```python
from build123d import *

# Parameters (mm, degrees)
SKETCH_1_W          = 42
SKETCH_1_H          = 8
SKETCH_1_R          = 2.35
EXTRUDE_1_DEPTH     = 32
SKETCH_2_W          = 23
SKETCH_2_H          = 20
CUT_EXTRUDE_2_DEPTH = 14
SKETCH_3_W          = 23
SKETCH_3_H          = 27.182471636
CUT_EXTRUDE_3_DEPTH = 10


with BuildPart() as part:
    # 草图1 → 凸台-拉伸1 (new, symmetric)
    with BuildSketch(Plane.XY):
        Rectangle(SKETCH_1_W, SKETCH_1_H)
        with Locations((-4.925, 0)):
            Circle(SKETCH_1_R, mode=Mode.SUBTRACT)
        with Locations(Location((4.925, 0, 0), (0, 0, 180))):
            Circle(SKETCH_1_R, mode=Mode.SUBTRACT)
        with Locations((-14.775, 0)):
            Circle(SKETCH_1_R, mode=Mode.SUBTRACT)
        with Locations(Location((14.775, 0, 0), (0, 0, 180))):
            Circle(SKETCH_1_R, mode=Mode.SUBTRACT)
    extrude(amount=EXTRUDE_1_DEPTH, both=True)

    # 草图2 → 切除-拉伸2 (cut)
    with BuildSketch(Plane(origin=(0, 4, 0), x_dir=(1, 0, 0), z_dir=(0, 1, 0))):
        with Locations((0, -15)):
            Rectangle(SKETCH_2_W, SKETCH_2_H)
        with Locations((0, 15)):
            Rectangle(SKETCH_2_W, SKETCH_2_H)
    extrude(amount=-CUT_EXTRUDE_2_DEPTH, mode=Mode.SUBTRACT)

    # 草图3 → 切除-拉伸3 (cut)
    with BuildSketch(Plane(origin=(0, 4, 0), x_dir=(1, 0, 0), z_dir=(0, 1, 0))):
        Rectangle(SKETCH_3_W, SKETCH_3_H)
    extrude(amount=-CUT_EXTRUDE_3_DEPTH, mode=Mode.SUBTRACT)


solid = part.part
```
The model under review builds one solid part; all positions refer to its coordinate system, in mm. A direction names the side the tool comes from. Coordinates: 2 decimals unless noted, no trailing zeros. Write each loop counter-clockwise with the first axis right and the second up, starting at its lowest first coordinate (ties: lowest second). Pieces come first, ordered by that corner, then holes. Notation, with made-up numbers: (79, 40) - (116, 40) arc R11 cw to (116, 60) - close; hole circle Ø7 at (66.5, 30.25). An arc over 180 degrees is marked (long way). Answer in a Markdown table with one row per item. Add a question column.
Q1. Draft analysis for pull direction Z (two halves, no side actions). For faces 3 (the face through (11.5, 0, 0)), 4 (the face through (0, 0, 32)), 5 (the face through (12.534, -0.706, -0.448)), state which applies: +Z half, -Z half, draft (parallel to the pull), parting line (faces both ways), or undercut.
Q2. Consider section D-D on y = 0. Give the number of separate pieces and of enclosed holes in the cut face, then the cut area to 3 significant figures.
Q3. Consider section C-C on y = -3. Give the boundary of the cut face in (x, z).
Q4. To check wall thickness, follow line 1 along X through (y, z) = (3, -9); line 2 along X through (y, z) = (-1.75, -26); line 3 along Z through (x, y) = (10.5, 3.5). State the ranges of each line that lie inside material, in increasing order. Write a range as from..to.
Q5. Consider section A-A on x = 8.5. Give the boundary of the cut face in (y, z), then the cut area to 3 significant figures.
Q6. Consider section B-B on z = 6.5. Give the boundary of the cut face in (x, y) (3 decimals), then the cut area to 3 significant figures.
Q7. For faces 1 (the face through (-5.4, -2.3, -28.5)), 2 (the face through (-11.5, 0, 0)), list the 3-axis set-ups (+Z, -Z, +X, -X, +Y, -Y) from which the entire face can be reached by the end or side of a thin tool; tool diameter is ignored.
Q8. Clearance check with a flat-ended pin moving along its axis: pin 1 (10 mm diameter, centred on x = -3.5, z = -17.5, fed in from -Y). State where the tip first meets the part, or that it passes through.
Answers below:
| question | item | result |
|---|---|---|
| 1 | face 3 | undercut |
| 1 | face 4 | +Z half |
| 1 | face 5 | draft |
| 2 | separate pieces | 6 |
| 2 | enclosed holes | 0 |
| 2 | area | 805 mm² |
| 3 | outline | (-21, -32) - (21, -32) - (21, 32) - (-21, 32) - close; hole (-11.5, -25) - (11.5, -25) - (11.5, 25) - (-11.5, 25) - close |
| 4 | line 1 | -21..-11.5, 11.5..21 |
| 4 | line 2 | -21..-16.34, -13.21..-6.49, -3.36..3.36, 6.49..13.21, 16.34..21 |
| 4 | line 3 | -32..-25, 25..32 |
| 5 | outline | (-4, -32) - (4, -32) - (4, -25) - (-4, -25) - close; (-4, 25) - (4, 25) - (4, 32) - (-4, 32) - close |
| 5 | area | 112 mm² |
| 6 | outline | (-21, -4) - (-11.5, -4) - (-11.5, 4) - (-21, 4) - close; (11.5, -4) - (21, -4) - (21, 4) - (11.5, 4) - close; hole circle Ø4.7 at (-14.775, 0); hole circle Ø4.7 at (14.775, 0) |
| 6 | area | 117 mm² |
| 7 | face 1 | +Z, -Z |
| 7 | face 2 | +Y, -Y |
| 8 | pin 1 | through |
